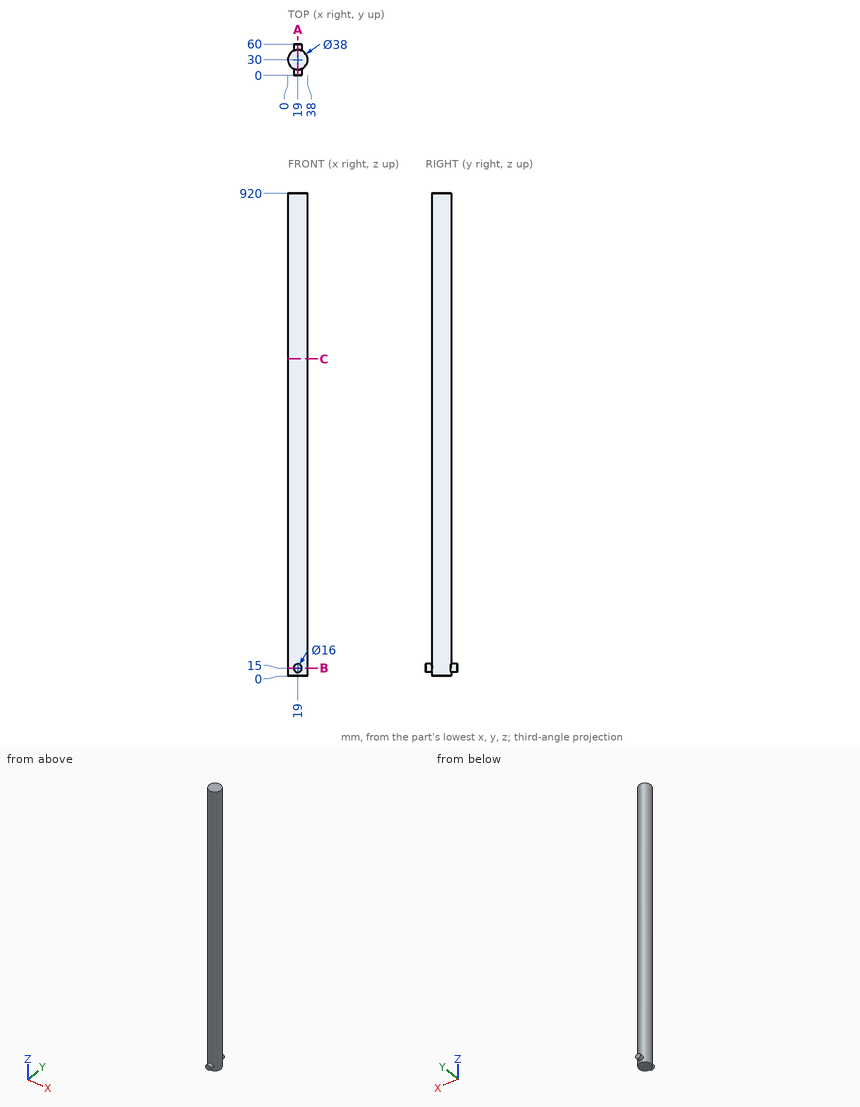
Print and shaded views of the part. All mm, measured from the part's lowest x, y and z. Coordinates: 2 decimals unless noted, no trailing zeros. Loops run counter-clockwise (first coordinate to the right, second up) from the corner with the lowest first, then second, coordinate; pieces in that order, holes last. Notation, with made-up numbers: M 87.5,-24 L 117.5,-24 A17 ccw 117.5,-16 Z; hole C -15.75,-25.5 d4. An arc over 180 degrees is marked long. Use a Markdown table: item, result. Add a question column.
Q1. Cut at A-A (x = 19). Write the cut outline in (y, z).
Q2. Cut at C-C (z = 604.5). Write the cut outline in (x, y).
Q3. Probe L1, parallel to Y at x = 17.5, z = 311; L2, parallel to X at y = 32, z = 41; L3, parallel to Z at x = 19, y = 6. List the from-to ranges inside material, lowest first.
Q4. Cut at B-B (z = 15). Write the cut outline in (x, y), and give its area (3 significant figures).
Q5. Pin check, flat tips, straight feed: P1, Ø4, axis at x = 7.5, z = 298, coming from the +Y side; P2, Ø2, axis at x = 23, z = 105.5, coming from the -Y side; P3, Ø2, axis at y = 40, z = 642, coming from the +X side. Stop position of each tip, or through.
Worked out:
| question | item | result |
|---|---|---|
| 1 | outline | M 0,7 L 11,7 L 11,0 L 49,0 L 49,7 L 60,7 L 60,23 L 49,23 L 49,920 L 11,920 L 11,23 L 0,23 Z |
| 2 | outline | C 19,30 d38 |
| 3 | L1 | y = 11.06 to 48.94 |
| 3 | L2 | x = 0.11 to 37.89 |
| 3 | L3 | z = 7 to 23 |
| 4 | outline | M 11,0 L 27,0 L 27,12.77 A19 ccw 27,47.23 L 27,60 L 11,60 L 11,47.23 A19 ccw 11,12.77 Z |
| 4 | area | 1,500 mm2 |
| 5 | P1 | stops at y = 46.45 |
| 5 | P2 | stops at y = 11.24 |
| 5 | P3 | stops at x = 35.73 |
